Can you work these out from the model? Positions are in its coordinate system, mm. A direction names the side the tool comes from. Coordinates: 2 decimals unless noted, no trailing zeros. Write each loop counter-clockwise with the first axis right and the second up, starting at its lowest first coordinate (ties: lowest second). Pieces come first, ordered by that corner, then holes.
```python
from build123d import *

# Parameters (mm, degrees)
F0_W     = 100
F0_H     = 100
F1_DEPTH = 15
F3_DEPTH = 25
F4_R     = 30
F5_DEPTH = 15.001
F6_W     = 20
F6_H     = 20
F7_DEPTH = 60


with BuildPart() as f1:
    # F0 (on Top) → F1 (new body)
    with BuildSketch(Plane.XY):
        Rectangle(F0_W, F0_H)
    extrude(amount=F1_DEPTH)

    # F2 (on face) → F3 (join)
    with BuildSketch(Plane.XY.offset(15)):
        Polygon((-30, 30), (50, 30), (50, 50), (-50, 50), (-50, -50), (-30, -50), align=None)
    extrude(amount=F3_DEPTH)

    # F4 (on face) → F5 (cut, through all)
    with BuildSketch(Plane.XY.offset(15)):
        with Locations((10, -10)):
            Circle(F4_R)
    extrude(amount=-F5_DEPTH, mode=Mode.SUBTRACT)

    # F6 (on face) → F7 (join)
    with BuildSketch(Plane.XY.offset(40)):
        with Locations((-40, 40)):
            Rectangle(F6_W, F6_H)
    extrude(amount=F7_DEPTH)


solid = f1.part
```
1. If we section it at C-C, the plane y = 37.5: List the corners of the cut face in (x, z) for me.
2. Which directions (+Z, -Z, +X, -X, +Y, -Y) give clear straight access to the entire face, cutting with the end or side of a thin tool? Please do faces 1 (the face through (-17, 8, 15)), 2 (the face through (-40, -9, 40)), 3 (the face through (9, 40, 40)), 4 (the face through (-50, 10, 27)).
3. I'm going to push flat-ended pins straight in: P1, Ø10, axis at x = -42.5, y = 6.5, coming from the +Z side; P2, Ø12.5, axis at y = -26, z = 33.5, coming from the +X side; P3, Ø16, axis at x = -38.5, z = 81, coming from the -Y side. Where does each tip first touch, or does it pass through?
4. If I drill on L1, parallel to Y at x = 10, z = 8.75; L2, parallel to Y at x = 26.5, z = 28.5; L3, parallel to X at y = 32.5, z = 83.5, over which ranges is the centre line in solid material (lowest first)?
5. We'd pull the mould along X, two halves only. Please class faces 5 (the face through (-19.97, -8.68, 7.6)), 6 (the face through (-30, 40, 70)), 7 (the face through (-12, 50, 27)): released by +X, released by -X, zero draft, split by the parting line, or undercut.
6. If we section it at A-A, the plane x = 10: List the corners of the cut face in (y, z) for me.
7. If we section it at B-B, the plane y = -10: List the corners of the cut face in (x, z) for me, plus the area to 3 significant figures.
8. If we section it at D-D, the plane z = 18.5: List the corners of the cut face in (x, y) for me, plus the area to 3 significant figures.
Answers:
1. outline: (-50, 0) - (50, 0) - (50, 40) - (-30, 40) - (-30, 100) - (-50, 100) - close
2. face 1: +Z, +X, -Y
2. face 2: +Z, +X, -X, -Y
2. face 3: +Z, +X, +Y, -Y
2. face 4: +Z, -Z, -X, +Y, -Y
3. P1: stops at z = 40
3. P2: stops at x = -30
3. P3: stops at y = 30
4. L1: y = -50 to -40, 20 to 50
4. L2: y = 30 to 50
4. L3: x = -50 to -30
5. face 5: undercut
5. face 6: released by +X
5. face 7: zero draft
6. outline: (-50, 0) - (-40, 0) - (-40, 15) - (-50, 15) - close; (20, 0) - (50, 0) - (50, 40) - (30, 40) - (30, 15) - (20, 15) - close
7. outline: (-50, 0) - (-20, 0) - (-20, 15) - (-30, 15) - (-30, 40) - (-50, 40) - close; (40, 0) - (50, 0) - (50, 15) - (40, 15) - close
7. area: 1,100 mm2
8. outline: (-50, -50) - (-30, -50) - (-30, 30) - (50, 30) - (50, 50) - (-50, 50) - close
8. area: 3,600 mm2
